Here's how the part is built. I have some questions about the finished solid (model axes, mm). A direction names the side the tool comes from. Round coordinates to 2 decimals unless told otherwise and drop trailing zeros. Write each loop counter-clockwise with the first axis right and the second up, starting at its lowest first coordinate (ties: lowest second). Pieces come first, ordered by that corner, then holes. Notation, with made-up numbers: (14, -27) -> (63, -27) arc R35 cw to (63, 5) -> close; hole circle Ø11 at (-5, -28.5). An arc over 180 degrees is marked (long way). Answer in a Markdown table with one row per item.
from build123d import *

# Parameters (mm, degrees)
SALIENTE_EXTRUIR1_DEPTH = 4
CROQUIS2_W              = 4
CROQUIS2_H              = 71
SALIENTE_EXTRUIR2_DEPTH = 125.5
CORTAR_EXTRUIR2_START   = 55.720628
CROQUIS3_R              = 3.5
CORTAR_EXTRUIR2_DEPTH   = 59.720627748
CROQUIS4_R              = 3
CORTAR_EXTRUIR3_DEPTH   = 4
CROQUIS5_R              = 12.25
CORTAR_EXTRUIR4_DEPTH   = 1


with BuildPart() as part:
    # Croquis1 → Saliente-Extruir1 (new body)
    with BuildSketch(Plane(origin=(0, 0, 0), x_dir=(1, 0, 0), z_dir=(0, 1, 0))):
        with BuildLine():
            Line((-29.779372252, -36), (40.220627748, -36))
            Line((40.220627748, -36), (40.220627748, -34))
            ThreePointArc((40.220627748, -34), (37.745754014, -28.025126266), (43.720627748, -30.5))
            Line((43.720627748, -30.5), (55.720627748, -30.5))
            Line((55.720627748, -30.5), (55.720627748, 29.5))
            Line((55.720627748, 29.5), (43.720627748, 29.5))
            ThreePointArc((43.720627748, 29.5), (37.745754014, 27.025126266), (40.220627748, 33))
            Line((40.220627748, 33), (40.220627748, 35))
            Line((40.220627748, 35), (-29.779372252, 35))
            Line((-29.779372252, 35), (-29.779372252, 33))
            ThreePointArc((-29.779372252, 33), (-27.304498518, 31.974873734), (-26.279372252, 29.5))
            ThreePointArc((-26.279372252, 29.5), (-29.779372252, 26), (-33.279372252, 29.5))
            Line((-33.279372252, 29.5), (-45.279372252, 29.5))
            Line((-45.279372252, 29.5), (-45.279372252, -30.5))
            Line((-45.279372252, -30.5), (-33.279372252, -30.5))
            ThreePointArc((-33.279372252, -30.5), (-29.779372252, -27), (-26.279372252, -30.5))
            ThreePointArc((-26.279372252, -30.5), (-27.304498518, -32.974873734), (-29.779372252, -34))
            Line((-29.779372252, -34), (-29.779372252, -36))
        make_face()
        with BuildLine():
            Line((-45.279372252, -36), (-29.779372252, -36))
            Line((-29.779372252, -36), (-29.779372252, -34))
            ThreePointArc((-29.779372252, -34), (-32.254245986, -32.974873734), (-33.279372252, -30.5))
            Line((-33.279372252, -30.5), (-45.279372252, -30.5))
            Line((-45.279372252, -30.5), (-45.279372252, -36))
        make_face()
        with BuildLine():
            Line((40.220627748, -34), (40.220627748, -36))
            Line((40.220627748, -36), (55.720627748, -36))
            Line((55.720627748, -36), (55.720627748, -30.5))
            Line((55.720627748, -30.5), (43.720627748, -30.5))
            ThreePointArc((43.720627748, -30.5), (42.695501482, -32.974873734), (40.220627748, -34))
        make_face()
        with BuildLine():
            Line((43.720627748, 29.5), (55.720627748, 29.5))
            Line((55.720627748, 29.5), (55.720627748, 35))
            Line((55.720627748, 35), (40.220627748, 35))
            Line((40.220627748, 35), (40.220627748, 33))
            ThreePointArc((40.220627748, 33), (42.695501482, 31.974873734), (43.720627748, 29.5))
        make_face()
        with BuildLine():
            Line((-45.279372252, 35), (-45.279372252, 29.5))
            Line((-45.279372252, 29.5), (-33.279372252, 29.5))
            ThreePointArc((-33.279372252, 29.5), (-32.254245986, 31.974873734), (-29.779372252, 33))
            Line((-29.779372252, 33), (-29.779372252, 35))
            Line((-29.779372252, 35), (-45.279372252, 35))
        make_face()
    extrude(amount=SALIENTE_EXTRUIR1_DEPTH)

    # Croquis2 → Saliente-Extruir2 (add)
    with BuildSketch(Plane(origin=(0, 0, 0), x_dir=(1, 0, 0), z_dir=(0, 1, 0))):
        with Locations((57.720627748, -0.5)):
            Rectangle(CROQUIS2_W, CROQUIS2_H)
    extrude(amount=SALIENTE_EXTRUIR2_DEPTH)

    # Croquis3 → Cortar-Extruir2 (cut)
    with BuildSketch(Plane(origin=(0, 0, 0), x_dir=(0, 0, -1), z_dir=(1, 0, 0)).offset(CORTAR_EXTRUIR2_START)):
        with BuildLine():
            ThreePointArc((29, 113.5), (26.878679656, 112.621320344), (26, 110.5))
            Line((26, 110.5), (35, 110.5))
            Line((35, 110.5), (35, 113.5))
            Line((35, 113.5), (29, 113.5))
        make_face()
        with BuildLine():
            ThreePointArc((26, 110.5), (26.878679656, 108.378679656), (29, 107.5))
            Line((29, 107.5), (35, 107.5))
            Line((35, 107.5), (35, 110.5))
            Line((35, 110.5), (26, 110.5))
        make_face()
        with BuildLine():
            Line((-36, 110.5), (-27, 110.5))
            ThreePointArc((-27, 110.5), (-27.878679656, 112.621320344), (-30, 113.5))
            Line((-30, 113.5), (-36, 113.5))
            Line((-36, 113.5), (-36, 110.5))
        make_face()
        with BuildLine():
            ThreePointArc((-30, 107.5), (-27.878679656, 108.378679656), (-27, 110.5))
            Line((-27, 110.5), (-36, 110.5))
            Line((-36, 110.5), (-36, 107.5))
            Line((-36, 107.5), (-30, 107.5))
        make_face()
        with Locations(Location((29.5, 20.5, 0), (0, 0, 180))):
            Circle(CROQUIS3_R)
        with Locations(Location((-30.5, 20.5, 0), (0, 0, 180))):
            Circle(CROQUIS3_R)
    extrude(amount=CORTAR_EXTRUIR2_DEPTH, mode=Mode.SUBTRACT)

    # Croquis4 → Cortar-Extruir3 (cut)
    with BuildSketch(Plane(origin=(0, 4, 0), x_dir=(1, 0, 0), z_dir=(0, 1, 0))):
        with Locations(Location((5.220627748, -0.5, 0), (0, 0, 270))):
            Circle(CROQUIS4_R)
    extrude(amount=-CORTAR_EXTRUIR3_DEPTH, mode=Mode.SUBTRACT)

    # Croquis5 → Cortar-Extruir4 (cut)
    with BuildSketch(Plane.XZ):
        with Locations(Location((5.220627748, 0.5, 0), (0, 0, 270))):
            Circle(CROQUIS5_R)
    extrude(amount=-CORTAR_EXTRUIR4_DEPTH, mode=Mode.SUBTRACT)


solid = part.part
1) I want a section at A-A, the plane y = 20.5. List the corners of the cut face in (x, z) for me.
Response:
| item | result |
|---|---|
| outline | (55.72, -35) -> (59.72, -35) -> (59.72, -33) -> (55.72, -33) -> close; (55.72, -26) -> (59.72, -26) -> (59.72, 27) -> (55.72, 27) -> close; (55.72, 34) -> (59.72, 34) -> (59.72, 36) -> (55.72, 36) -> close |
2) I want a section at D-D, the plane x = -3. List the corners of the cut face in (y, z) for me.
Response:
| item | result |
|---|---|
| outline | (0, -35) -> (4, -35) -> (4, 36) -> (0, 36) -> (0, 9.58) -> (1, 9.58) -> (1, -8.58) -> (0, -8.58) -> close |
3) I want a section at B-B, the plane z = 0.5. List the corners of the cut face in (x, y) for me, and give its area (4 significant figures).
Response:
| item | result |
|---|---|
| outline | (-45.28, 0) -> (-7.03, 0) -> (-7.03, 1) -> (2.22, 1) -> (2.22, 4) -> (-45.28, 4) -> close; (8.22, 1) -> (17.47, 1) -> (17.47, 0) -> (59.72, 0) -> (59.72, 125.5) -> (55.72, 125.5) -> (55.72, 4) -> (8.22, 4) -> close |
| area | 863.5 mm^2 |
4) I need wall thicknesses on line 1 (Y direction, x = 56, z = 30); line 2 (Z direction, x = 56, y = 20); line 3 (X direction, y = 3, z = 30.5). Which ranges of each line are inside material? Lowest first, please. Write a range as [from, to].
Response:
| item | result |
|---|---|
| line 1 | y = [0, 17.04], [23.96, 107.5], [113.5, 125.5] |
| line 2 | z = [-35, -32.96], [-26.04, 27.04], [33.96, 36] |
| line 3 | x = [-45.28, -33.28], [-26.28, 36.72], [43.72, 59.72] |
5) We'd pull the mould along Z, two halves only. Please class faces 1 (the face through (58, 113.5, 33)), 2 (the face through (58, 119, -35)), 3 (the face through (57.69, 17.55, -27.62)), 4 (the face through (3, 1, -2)): +Z half, -Z half, draft (parallel to the pull), parting line (faces both ways), or undercut.
Response:
| item | result |
|---|---|
| face 1 | draft |
| face 2 | -Z half |
| face 3 | undercut |
| face 4 | undercut |
6) Which directions (+Z, -Z, +X, -X, +Y, -Y) give clear straight access to the entire face, cutting with the end or side of a thin tool? Please do faces 5 (the face through (58, 113.5, -32)), 6 (the face through (8.9, 0.493, -11.184)), 7 (the face through (58, 107.5, 33)), 8 (the face through (5, 4, -8)).
Response:
| item | result |
|---|---|
| face 5 | -Z, +X, -X |
| face 6 | -Y |
| face 7 | +Z, +X, -X |
| face 8 | +Z, -Z, -X, +Y |
7) For pin 1 (7.5 mm diameter, centred on x = 8, z = -1.5, fed in from -Y); pin 2 (1 mm diameter, centred on x = -19, z = 9, fed in from +Y); pin 3 (1.5 mm diameter, centred on y = 98.5, z = 11, fed in from -X); pin 4 (4 mm diameter, centred on x = 46, z = -27.5, fed in from -Y), each with a flat end and sliding along its axis, tell me the tip position at first contact or that it passes through.
Response:
| item | result |
|---|---|
| pin 1 | stops at y = 1 |
| pin 2 | stops at y = 4 |
| pin 3 | stops at x = 55.72 |
| pin 4 | stops at y = 0 |
8) I want a section at C-C, the plane z = 16. List the corners of the cut face in (x, y) for me.
Response:
| item | result |
|---|---|
| outline | (-45.28, 0) -> (59.72, 0) -> (59.72, 125.5) -> (55.72, 125.5) -> (55.72, 4) -> (-45.28, 4) -> close |
